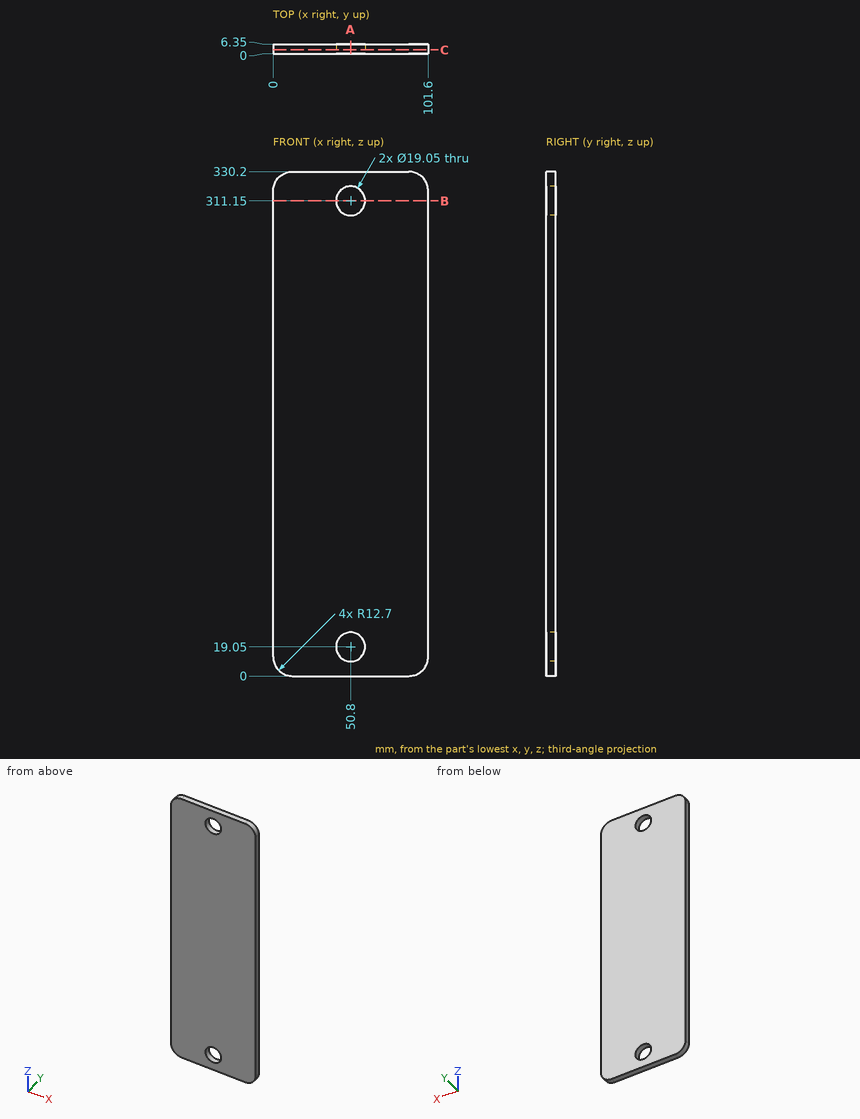
Geometry: see drawing. Coordinates: mm, zero at the bounding-box minimum. Round coordinates to 2 decimals unless told otherwise and drop trailing zeros. Order: outer loops, then holes, each group sorted by start corner. A loop starts at its lowest first (then second) coordinate and runs counter-clockwise, first axis right, second up. Notation, with made-up numbers: (-0.5, -38.75) -> (55.5, -38.75) arc R25 cw to (55.5, -21.75) -> close; hole circle Ø9 at (80, 8). An arc over 180 degrees is marked (long way). Write each question's results on one line, items separated by ' | '.
Q1. Section query C-C (y = 2.5). Output: boundary loops of the cut face in (x, z) (3 decimals).
Response values:
outline: (0, 12.7) arc R12.7 ccw to (12.7, 0) -> (88.9, 0) arc R12.7 ccw to (101.6, 12.7) -> (101.6, 317.5) arc R12.7 ccw to (88.9, 330.2) -> (12.7, 330.2) arc R12.7 ccw to (0, 317.5) -> close; hole circle Ø19.05 at (50.8, 19.05); hole circle Ø19.05 at (50.8, 311.15)
Q2. Ray query, line 1 along Z through (x, y) = (50.8, 3) (3 decimals); line 2 along X through (y, z) = (5.5, 17.5); line 3 along Z through (x, y) = (56, 4). Return the intervals inside material, ascending.
Response values:
line 1: 0 to 9.525, 28.575 to 301.625, 320.675 to 330.2 | line 2: 0 to 41.4, 60.2 to 101.6 | line 3: 0 to 11.07, 27.03 to 303.17, 319.13 to 330.2
Q3. Section query A-A (x = 50.8). Output: boundary loops of the cut face in (y, z) (3 decimals), and give its area (3 significant figures).
Response values:
outline: (0, 0) -> (6.35, 0) -> (6.35, 9.525) -> (0, 9.525) -> close; (0, 28.575) -> (6.35, 28.575) -> (6.35, 301.625) -> (0, 301.625) -> close; (0, 320.675) -> (6.35, 320.675) -> (6.35, 330.2) -> (0, 330.2) -> close | area: 1,850 mm²
Q4. Section query B-B (z = 311.15). Output: boundary loops of the cut face in (x, y) (3 decimals), and give its area (3 significant figures).
Response values:
outline: (0, 0) -> (41.275, 0) -> (41.275, 6.35) -> (0, 6.35) -> close; (60.325, 0) -> (101.6, 0) -> (101.6, 6.35) -> (60.325, 6.35) -> close | area: 524 mm²
